Read the model definition and answer for the solid it produces. Units are mm, in the model's axes. Coordinates: 2 decimals unless noted, no trailing zeros. Order: outer loops, then holes, each group sorted by start corner. A loop starts at its lowest first (then second) coordinate and runs counter-clockwise, first axis right, second up. Notation, with made-up numbers: (-30, 43) - (-25, 43) arc R34 cw to (-25, 74) - close; hole circle Ø3 at (7, 14). An arc over 180 degrees is marked (long way). Use one line per item in the form item = value.
```python
from build123d import *

# Parameters (mm, degrees)
SKETCH2_W = 0.6
SKETCH2_H = 0.6


with BuildPart() as part:
    # Sweep1: sweep along a path in Sketch1
    with BuildLine(Plane(origin=(0, 0, 0), x_dir=(0, 0, -1), z_dir=(1, 0, 0))) as sweep1_path:
        Line((5, -10.2), (-2.15, -10.2))
        ThreePointArc((-2.15, -10.2), (-2.397487373, -10.097487373), (-2.5, -9.85))
        Line((-2.5, -9.85), (-2.5, -1.5))
        ThreePointArc((-2.5, -1.5), (-2.060660172, -0.439339828), (-1, 0))
        Line((-1, 0), (0, 0))
    # Sketch2 → Sweep1 (sweep)
    with BuildSketch(Plane.XY):
        Rectangle(SKETCH2_W, SKETCH2_H)
    sweep(path=sweep1_path.line)


solid = part.part
```
(1) Section D-D, the plane z = -3.25 is taken. Write down the section's boundary in (x, y), then the cut area to 3 significant figures.
Answer list:
outline = (-0.3, -10.5) - (0.3, -10.5) - (0.3, -9.9) - (-0.3, -9.9) - close
area = 0.360 mm2
(2) Straight lines are drawn through the part: L1, parallel to Y at x = -0.2, z = -2.75; L2, parallel to Z at x = 0.25, y = -9; L3, parallel to Y at x = 0.2, z = 1.75. For each, find the intervals that lie inside material, in ascending order.
Answer list:
L1 = -10.5 to -9.9
L2 = 2.2 to 2.8
L3 = -10.5 to -9.9, -0.56 to 0.14
(3) Section C-C, the plane y = -4.5 is taken. Write down the section's boundary in (x, z).
Answer list:
outline = (-0.3, 2.2) - (0.3, 2.2) - (0.3, 2.8) - (-0.3, 2.8) - close
(4) Section A-A, the plane z = 0.25 is taken. Write down the section's boundary in (x, y).
Answer list:
outline = (-0.3, -10.5) - (0.3, -10.5) - (0.3, -9.9) - (-0.3, -9.9) - close; (-0.3, -0.3) - (0.3, -0.3) - (0.3, 0.3) - (-0.3, 0.3) - close
(5) Section B-B, the plane x = -0.1 is taken. Write down the section's boundary in (y, z).
Answer list:
outline = (-10.5, -5) - (-9.9, -5) - (-9.9, 2.15) arc R0.05 cw to (-9.85, 2.2) - (-1.5, 2.2) arc R1.2 cw to (-0.3, 1) - (-0.3, 0) - (0.3, 0) - (0.3, 1) arc R1.8 ccw to (-1.5, 2.8) - (-9.85, 2.8) arc R0.65 ccw to (-10.5, 2.15) - close
(6) The mould has two halves that part along Y. Classify faces 1 (the cylindrical face through (0.004, -0.661, 1.858)), 2 (the cylindrical face through (-0.004, -0.241, 2.287)), 3 (the flat face through (0.3, -5.9, 2.4)): +Y half, -Y half, draft (parallel to the pull), parting line (faces both ways), or undercut.
Answer list:
face_1 = undercut
face_2 = +Y half
face_3 = draft
(7) Given pin 1 Ø1.5 at (y, z) = (-9, 1) entering from +X, flat-ended and moving along its own axis, determine where the tip first touches the part or whether it passes through.
Answer list:
pin_1 = through
